Autodesk Inventor part; units mm, degrees
ref_plane "YZ Plane" through (0, 0, 0) normal (1, 0, 0) x (0, 1, 0)
ref_plane "XZ Plane" through (0, 0, 0) normal (0, 1, 0) x (-1, 0, 0)
ref_plane "XY Plane" through (0, 0, 0) normal (0, 0, 1) x (1, 0, 0)
sketch "Sketch1" plane through (0, 0, 0) normal (0, 0, 1) x (1, 0, 0)
  line L0 (0, 0) -> (0, 32.5)
  line L1 (0, 32.5) -> (13, 32.5)
  line L2 (13, 32.5) -> (13, 48.5)
  line L3 (13, 48.5) -> (24.3, 48.5)
  line L4 (24.3, 48.5) -> (24.3, 31.5)
  line L5 (24.3, 31.5) -> (46.9, 31.5)
  line L6 (46.9, 31.5) -> (46.9, 0)
  line L7 (0, 0) -> (46.9, 0)
  dimension "d0" = 32.5
  dimension "d1" = 13
  dimension "d2" = 16
  dimension "d3" = 11.3
  dimension "d4" = 17
  dimension "d5" = 22.6
revolve "Revolution1" add sketch "Sketch1" angle 360 about axis through (0, 0, 0) along (1, 0, 0)
sketch "Sketch2" plane through (13, 0, 0) normal (-1, 0, 0) x (0, 0, 1)
  circle A0 centre (0, 0) radius 32.5
  circle A1 centre (0, 0) radius 48.5
  circle A2 centre (0, 40.5) radius 3.5
  circle A3 centre (35.074, -20.25) radius 3.5
  circle A4 centre (-35.074, -20.25) radius 3.5
  dimension "d11" = 7
  dimension "d12" = 7
  dimension "d13" = 7
extrude "Extrusion1" cut sketch "Sketch2" against normal through all contours A2 | A3 | A4
sketch "Sketch3" plane through (0, 0, 0) normal (-1, 0, 0) x (0, 0, 1)
  circle A0 centre (0, 0) radius 17.5
  dimension "d16" = 35
sketch "Sketch4" plane through (0, 0, 0) normal (-1, 0, 0) x (0, 0, 1)
  point P0 (0, 0)
extrude "Extrusion2" cut sketch "Sketch3" against normal through all
sketch "Sketch5" plane through (46.9, 0, 0) normal (1, 0, 0) x (0, 0, -1)
  circle A0 centre (0, 0) radius 31.5
  circle A1 centre (0, 0) radius 26.2
extrude "Extrusion3" cut sketch "Sketch5" against normal blind 22.5 contours A1
properties part number "capa da engrenagem"
Part model, mm, in its own coordinate system. A direction names the side the tool comes from. Give positions to 0.01 mm unless a question says otherwise; leave off trailing zeros. Order: outer loops, then holes, each group sorted by start corner. A loop starts at its lowest first (then second) coordinate and runs counter-clockwise, first axis right, second up. Notation, with made-up numbers: M 21.5,-33 L 58.5,-33 A16 ccw 58.5,-25 Z; hole C -34,5 d7. An arc over 180 degrees is marked long. Use a Markdown table: item, result. Add a question column.
(1) Saw through at D-D, the plane x = 41.5. Give the cut face in (y, z), and give its area (3 significant figures).
(2) Saw through at C-C, the plane x = 15.5. Give the cut face in (y, z), and give its area (3 significant figures).
(3) 3-axis set-ups, long thin cutter, end or side, ignore diameter. For faces 1 (the face through (35.808, 25.977, 3.411)), 2 (the face through (12.029, -10.648, -13.887)), 3 (the face through (13, 10, -32)): which of +Z, -Z, +X, -X, +Y, -Y reach the whole face in a straight line?
(4) Drop flat-ended pins along their axis: P1, Ø1, axis at x = 8.5, z = -18, coming from the -Y side; P2, Ø1, axis at x = 10.5, z = -19.5, coming from the +Y side; P3, Ø6, axis at x = 37, z = 19, coming from the +Y side; P4, Ø2, axis at y = 33.5, z = -37.5, coming from the +X side. Give the stop position or say it passes through.
(5) Probe line 1 along Z through (x, y) = (12.5, 1); line 2 along Z through (x, y) = (18, -20); line 3 along Y through (x, z) = (26.5, -0.5). List the from-to ranges inside material, lowest first. Write a range as [from, to].
(6) Mould opens along Y. For faces 4 (the face through (24.4, -5, -17)), 5 (the face through (6.59, 31, 9.76)), 6 (the face through (0, 14, -14)), 7 (the face through (19, 44, 0)) say: +Y half, -Y half, draft (parallel to the pull), parting line (faces both ways), or undercut.
(7) Saw through at B-B, the plane y = 12.5. Give the cut face in (x, z).
(8) Saw through at A-A, the plane z = 0. Give the cut face in (x, y).
Answer key:
| question | item | result |
|---|---|---|
| 1 | outline | C 0,0 d63; hole C 0,0 d52.4 |
| 1 | area | 961 mm^2 |
| 2 | outline | C 0,0 d97; hole C -20.25,-35.07 d7; hole C -20.25,35.07 d7; hole C 0,0 d35; hole C 40.5,0 d7 |
| 2 | area | 6,310 mm^2 |
| 3 | face 1 | +X |
| 3 | face 2 | +X, -X |
| 3 | face 3 | -X |
| 4 | P1 | y = -27.39 |
| 4 | P2 | y = 26.37 |
| 4 | P3 | y = 27.13 |
| 4 | P4 | through |
| 5 | line 1 | [-32.48, -17.47], [17.47, 32.48] |
| 5 | line 2 | [-44.18, -38.57], [-31.58, 31.58], [38.57, 44.18] |
| 5 | line 3 | [-31.5, -26.2], [26.2, 31.5] |
| 6 | face 4 | undercut |
| 6 | face 5 | parting line |
| 6 | face 6 | draft |
| 6 | face 7 | undercut |
| 7 | outline | M 0,-30 L 13,-30 L 13,-46.86 L 24.3,-46.86 L 24.3,-28.91 L 46.9,-28.91 L 46.9,-23.03 L 24.4,-23.03 L 24.4,-12.25 L 0,-12.25 Z; M 0,12.25 L 24.4,12.25 L 24.4,23.03 L 46.9,23.03 L 46.9,28.91 L 24.3,28.91 L 24.3,46.86 L 13,46.86 L 13,30 L 0,30 Z |
| 8 | outline | M 0,-32.5 L 13,-32.5 L 13,-48.5 L 24.3,-48.5 L 24.3,-31.5 L 46.9,-31.5 L 46.9,-26.2 L 24.4,-26.2 L 24.4,-17.5 L 0,-17.5 Z; M 0,17.5 L 24.4,17.5 L 24.4,26.2 L 46.9,26.2 L 46.9,31.5 L 24.3,31.5 L 24.3,37 L 13,37 L 13,32.5 L 0,32.5 Z; M 13,44 L 24.3,44 L 24.3,48.5 L 13,48.5 Z |
